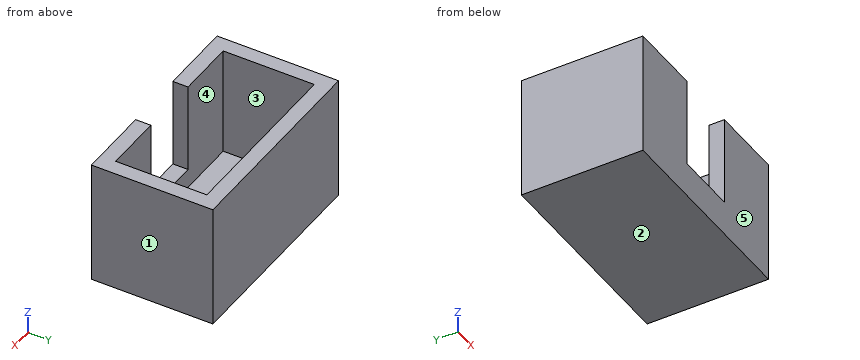
```python
from build123d import *

# Parameters (mm, degrees)
F0_W     = 15.2
F0_H     = 8.8
F1_DEPTH = 9
F2_T     = -1.1
F3_W     = 4.5
F3_H     = 6.5
F4_DEPTH = 1.1


with BuildPart() as f1:
    # F0 (on Top) → F1 (new body)
    with BuildSketch(Plane.XY):
        with Locations((7.6, 4.4)):
            Rectangle(F0_W, F0_H)
    extrude(amount=F1_DEPTH)

    # F2
    f2_openings = [f1.faces().sort_by_distance(p)[0] for p in [
        (7.6, 4.4, 9),
    ]]
    offset(amount=F2_T, openings=f2_openings)

    # F3 (on face) → F4 (cut, through all)
    with BuildSketch(Plane.XZ):
        with Locations((7.6, 5.75)):
            Rectangle(F3_W, F3_H)
    extrude(amount=-F4_DEPTH, mode=Mode.SUBTRACT)


solid = f1.part
```
Here's how the part is built. I have some questions about the finished solid (model axes, mm). Face numbers are marked on the shaded views. A direction names the side the tool comes from. Round coordinates to 2 decimals unless told otherwise and drop trailing zeros. Order: outer loops, then holes, each group sorted by start corner. A loop starts at its lowest first (then second) coordinate and runs counter-clockwise, first axis right, second up. Notation, with made-up numbers: M 76,32 L 131,32 A29 ccw 131,65 Z; hole C -0.75,79.5 d6. An arc over 180 degrees is marked long. Use CSV: the item, a comma, the result in double quotes.
1) I want a section at D-D (y = 6.5). List the corners of the cut face in (x, z) for me, then the cut area to 3 significant figures.
Taken from the geometry:
outline,"M 0,0 L 15.2,0 L 15.2,9 L 14.1,9 L 14.1,1.1 L 1.1,1.1 L 1.1,9 L 0,9 Z"
area,"34.1 mm^2"
2) I need wall thicknesses on line 1 along X through (y, z) = (2, 7.25); line 2 along Y through (x, z) = (2, 4); line 3 along Z through (x, y) = (6, 7.25). Which ranges of each line are inside material? Lowest first, please. Write a range as [from, to].
Taken from the geometry:
line 1,"[0, 1.1], [14.1, 15.2]"
line 2,"[0, 1.1], [7.7, 8.8]"
line 3,"[0, 1.1]"
3) I want a section at B-B (x = 9.5). List the corners of the cut face in (y, z) for me, then the cut area to 3 significant figures.
Taken from the geometry:
outline,"M 0,0 L 8.8,0 L 8.8,9 L 7.7,9 L 7.7,1.1 L 1.1,1.1 L 1.1,2.5 L 0,2.5 Z"
area,"19.9 mm^2"
4) If we mould it in two halves opening along X, with no side actions, what happens to the marked faces 1, 2 and 3? For each: pulls with the +X half, pulls with the -X half, needs draft (parallel to the pull), parting line crosses it, or undercut.
Taken from the geometry:
face 1,"pulls with the +X half"
face 2,"needs draft"
face 3,"undercut"
5) I want a section at A-A (z = 1.75). List the corners of the cut face in (x, y) for me, then the cut area to 3 significant figures.
Taken from the geometry:
outline,"M 0,0 L 15.2,0 L 15.2,8.8 L 0,8.8 Z; hole M 1.1,1.1 L 14.1,1.1 L 14.1,7.7 L 1.1,7.7 Z"
area,"48.0 mm^2"
6) I want a section at C-C (z = 3.25). List the corners of the cut face in (x, y) for me, then the cut area to 3 significant figures.
Taken from the geometry:
outline,"M 0,0 L 5.35,0 L 5.35,1.1 L 1.1,1.1 L 1.1,7.7 L 14.1,7.7 L 14.1,1.1 L 9.85,1.1 L 9.85,0 L 15.2,0 L 15.2,8.8 L 0,8.8 Z"
area,"43.0 mm^2"
7) I'm going to push flat-ended pins straight in: P1, Ø2, axis at x = 10, y = 3, coming from the +Z side; P2, Ø3.5, axis at y = 3.5, z = 5, coming from the -X side; P3, Ø1.2, axis at x = 6.5, y = 0.5, coming from the +Z side. Where does each tip first touch, or does it pass through?
Taken from the geometry:
P1,"z = 1.1"
P2,"x = 0"
P3,"z = 2.5"
8) On a 3-axis mill with a long thin cutter (end or side, diameter ignored), from which of +Z, -Z, +X, -X, +Y, -Y can I reach the whole of each face in a straight line? I mean the marked faces 4 and 5. Say none if no direction works.
Taken from the geometry:
face 4,"+Z"
face 5,"+Z, -Z, +X, -X, -Y"
